Source: CAD feature listing. Evaluate the final solid. Frame: model axes, mm. A direction names the side the tool comes from. Coordinates: 2 decimals unless noted, no trailing zeros. Order: outer loops, then holes, each group sorted by start corner. A loop starts at its lowest first (then second) coordinate and runs counter-clockwise, first axis right, second up. Notation, with made-up numbers: (-27, -30) -> (-8, -30) arc R17 ccw to (-8, -7) -> close; hole circle Ø1 at (28.5, -35.5). An arc over 180 degrees is marked (long way). Write each question's results on one line, items separated by ' | '. Start each with the question number.
Autodesk Inventor part; units mm, degrees
ref_plane "YZ Plane" through (0, 0, 0) normal (1, 0, 0) x (0, 1, 0)
ref_plane "XZ Plane" through (0, 0, 0) normal (0, 1, 0) x (-1, 0, 0)
ref_plane "XY Plane" through (0, 0, 0) normal (0, 0, 1) x (1, 0, 0)
sketch "Sketch1" plane through (0, 0, 0) normal (0, 0, 1) x (1, 0, 0)
  line L0 (0, 0) -> (25, 0)
  line L1 (25, 0) -> (25, 40)
  line L2 (25, 40) -> (0, 40)
  line L3 (0, 40) -> (0, 0)
  dimension "d1" = 25
  dimension "d2" = 40
  dimension "d3" = 25
extrude "Extrusion1" add sketch "Sketch1" against normal blind 30
sketch "Sketch2" plane through (25, 0, 0) normal (1, 0, 0) x (0, 0, -1)
  line L0 (0, 0) -> (30, 0)
  circle A0 centre (15, 6.56) radius 2.46
extrude "Extrusion2" cut sketch "Sketch2" against normal blind 30
sketch "Sketch3" plane through (0, 0, 0) normal (-1, 0, 0) x (0, 0, 1)
  line L0 (0, 0) -> (-30, 0)
  line L1 (-25.05, 0) -> (-4.95, 0)
  line L2 (-4.95, 0) -> (-4.95, 33.12)
  line L3 (-4.95, 33.12) -> (-25.05, 33.12)
  line L4 (-25.05, 33.12) -> (-25.05, 0)
  dimension "d11" = 20.1
extrude "Extrusion3" cut sketch "Sketch3" against normal blind 20
sketch "Sketch4" plane through (0, 0, 0) normal (0, -1, 0) x (1, 0, 0)
  line L0 (20, -4.95) -> (20, -25.05)
  line L1 (20, -15) -> (25, -15)
  line L2 (25, 0) -> (25, -30)
  line L3 (20, -8.025) -> (25, -8.025)
  line L4 (25, -8.025) -> (25, -21.975)
  line L5 (25, -21.975) -> (20, -21.975)
  line L6 (20, -21.975) -> (20, -8.025)
  line L7 (20, -8.025) -> (25, -21.975) construction
  line L8 (25, -8.025) -> (20, -21.975) construction
  line L9 (25, -12.54) -> (25, -17.46)
  point P0 (0, 0)
  point P1 (22.5, -15)
  dimension "d14" = 13.95
extrude "Extrusion4" add sketch "Sketch4" along normal blind 15
sketch "Sketch5" plane through (20, 0, 0) normal (-1, 0, 0) x (0, 0, 1)
  circle A0 centre (-15, 6.56) radius 2.46
  circle A1 centre (-15, 6.56) radius 4.7025
  circle A2 centre (-15, 6.56) radius 2.46
  circle A3 centre (-15, 6.56) radius 2.46
  point P0 (0, 0)
  dimension "d17" = 9.405
extrude "Extrusion5" cut sketch "Sketch5" against normal blind 2.1
sketch "Sketch6" plane through (25, 0, 0) normal (1, 0, 0) x (0, 0, -1)
  circle A0 centre (15, 6.56) radius 4.7025
  line L0 (15, 6.56) -> (15, 23.56)
  circle A1 centre (15, 23.56) radius 2.46
  point P0 (0, 0)
  dimension "d20" = 17
  dimension "d21" = 4.92
extrude "Extrusion6" cut sketch "Sketch6" against normal blind 10 contours A1
sketch "Sketch7" plane through (20, 0, 0) normal (-1, 0, 0) x (0, 0, 1)
  circle A0 centre (-15, 23.56) radius 2.46
  circle A1 centre (-15, 23.56) radius 4.7025
  point P0 (0, 0)
  dimension "d24" = 9.405
extrude "Extrusion7" cut sketch "Sketch7" against normal blind 2.1
sketch "Sketch9" plane through (25, 0, 0) normal (1, 0, 0) x (0, 0, -1)
  circle A0 centre (15, 6.56) radius 2.46
  circle A1 centre (15, 6.56) radius 2.46
  circle A2 centre (15, 23.56) radius 2.46
  circle A3 centre (15, 23.56) radius 2.46
  line L0 (30, 40) -> (30, 0)
  line L1 (30, 0) -> (30, 40)
  line L2 (30, 40) -> (0, 40)
  line L3 (0, 40) -> (0, 0)
  line L4 (0, 0) -> (8.025, 0)
  line L5 (21.975, 0) -> (21.975, -15)
  line L6 (21.975, -15) -> (8.025, -15)
  line L7 (8.025, -15) -> (8.025, 0)
  line L8 (0, 0) -> (8.025, 0)
  line L9 (21.975, 0) -> (30, 0)
extrude "Extrusion8" add sketch "Sketch9" along normal blind 5
sketch "Sketch10" plane through (0, 40, 0) normal (0, 1, 0) x (1, 0, 0)
  line L0 (0, 30) -> (30, 30)
  line L1 (30, 0) -> (0, 0)
  line L2 (0, 30) -> (30, 30)
  line L3 (30, 30) -> (30, 0)
  line L4 (30, 0) -> (0, 0)
  line L5 (0, 0) -> (0, 30)
extrude "Extrusion9" add sketch "Sketch10" along normal blind 30
sketch "Sketch12" plane through (30, 0, 0) normal (1, 0, 0) x (0, 0, -1)
  circle A0 centre (15, 6.56) radius 2.46
  line L0 (15, 6.56) -> (15, 15.06)
  circle A1 centre (15, 15.06) radius 2.525
  point P0 (0, 0)
  dimension "d31" = 8.5
  dimension "d33" = 5.05
extrude "Extrusion10" cut sketch "Sketch12" against normal blind 30 contours A1
sketch "Sketch14" plane through (0, 0, 0) normal (0, 0, 1) x (1, 0, 0)
  line L0 (30, 70) -> (0, 70)
  line L1 (0, 70) -> (0, 85)
  line L2 (-15, 100) -> (-23, 100)
  line L3 (30, 0) -> (30, 70)
  line L4 (30, 113) -> (30, 70)
  arc A0 (0, 85) -> (-15, 100) centre (-15, 85) ccw
  line L5 (30, 105) -> (30, 100)
  line L6 (-23, 128) -> (15, 128)
  line L7 (30, 113) -> (15, 128)
  line L8 (-23, 128) -> (-23, 100)
  point P0 (0, 0)
  point P1 (0, 100)
  dimension "d47" = 30
  dimension "d54" = 15
  dimension "d69" = 28
extrude "Extrusion12" add sketch "Sketch14" against normal blind 30
sketch "Sketch15" plane through (0, 0, -25.05) normal (-1, 0, 0) x (0, 0, 1)
  line L0 (0, 33.12) -> (20.1, 33.12)
  line L1 (20.1, 33.12) -> (20.1, 0)
  line L2 (0, 33.12) -> (20.1, 33.12)
  line L3 (20.1, 33.12) -> (20.1, 31.1)
  line L4 (20.1, 31.1) -> (0, 31.1)
  line L5 (0, 31.1) -> (0, 33.12)
  point P0 (25.05, 0)
  dimension "d57" = 2.02
extrude "Extrusion13" add sketch "Sketch15" against normal blind 20
sketch "Sketch25" plane through (-23, 128, 0) normal (0, 1, 0) x (1, 0, 0)
  line L0 (0, 0) -> (0, 30)
  line L1 (8, 15) -> (0, 0)
  line L2 (8, 15) -> (0, 30)
  line L3 (8, 30) -> (0, 30)
  line L4 (0, 30) -> (0, 0)
  point P0 (23, 0)
extrude "Extrusion17" cut sketch "Sketch25" against normal through all
properties part number "orien_b_25mm"
(1) Section A-A on y = 6.56. Return the cut outline in (x, z).
(2) Section D-D on y = 39.5. Return the cut outline in (x, z).
(3) Line query: L1, parallel to Y at x = 21, z = -15 (1 decimal); L2, parallel to Z at x = 26, y = 23.56; L3, parallel to X at y = 15.5, z = -6. Output: solid intervals per line, ascending.
(4) Reachability of faces 5 (the flat face through (0, 53, -15)), 6 (the flat face through (25, -8, -8.025)), 7 (the flat face through (-18.944, 114.196, -22.395)), 8 (the flat face through (18, 0, -27)) from +Z, -Z, +X, -X, +Y, -Y: full face, straight path, thin tool, end or side. Return the list, or none.
(5) Section B-B on z = -28. Return the cut outline in (x, y), then the cut area to 3 significant figures.
(6) First-contact query: P1, Ø6, axis at y = -2, z = -17.5, coming from the -X side; P2, Ø8.5, axis at y = 23.56, z = -15, coming from the -X side; P3, Ø4, axis at x = 9.5, z = -2.5, coming from the -Y side; P4, Ø5.5, axis at y = 6.56, z = -15, coming from the +X side. Flat tips, straight axial feed; report the tip coordinate or a pass-through.
(7) Section C-C on x = -3. Return the cut outline in (y, z), then the cut area to 3 significant figures.
(8) Draft query along Z for faces 1 (the flat face through (10, 15, -4.95)), 2 (the flat face through (9, 65, 0)), 3 (the flat face through (-18.944, 114.196, -7.605)), 4 (the flat face through (30, 50, -15)). Return one class per face: released by +Z, released by -Z, zero draft, split by the parting line, or undercut.
Results list:
1) outline: (0, -30) -> (30, -30) -> (30, -17.46) -> (22.1, -17.46) -> (22.1, -19.7) -> (20, -19.7) -> (20, -25.05) -> (0, -25.05) -> close; (0, -4.95) -> (20, -4.95) -> (20, -10.3) -> (22.1, -10.3) -> (22.1, -12.54) -> (30, -12.54) -> (30, 0) -> (0, 0) -> close
2) outline: (0, -30) -> (30, -30) -> (30, 0) -> (0, 0) -> close
3) L1: y = -15 to 1.9, 11.3 to 12.5, 17.6 to 18.9, 28.3 to 122 | L2: z = -30 to -17.46, -12.54 to 0 | L3: x = 20 to 30
4) face 5: +Z, -Z, -X, -Y | face 6: +Z, +X, -X, -Y | face 7: -X, +Y, -Y | face 8: -Z, +X, -X, -Y
5) outline: (-21.93, 100) -> (-15, 100) arc R15 cw to (0, 85) -> (0, 0) -> (30, 0) -> (30, 113) -> (15, 128) -> (-21.93, 128) -> close | area: 4,390 mm²
6) P1: stops at x = 20 | P2: stops at x = 22.1 | P3: stops at y = 0 | P4: stops at x = 30
7) outline: (94, -30) -> (128, -30) -> (128, 0) -> (94, 0) -> close | area: 1,020 mm²
8) face 1: undercut | face 2: released by +Z | face 3: undercut | face 4: zero draft
